Here's the drawing with two shaded views (mm, measured from the low corner). I have some questions. A direction names the side the tool comes from. Coordinates: 2 decimals unless noted, no trailing zeros. Write each loop counter-clockwise with the first axis right and the second up, starting at its lowest first coordinate (ties: lowest second). Pieces come first, ordered by that corner, then holes. Notation, with made-up numbers: (85, 27) -> (138, 27) arc R11 ccw to (138, 47) -> close; hole circle Ø1 at (43.5, 83.25). An arc over 180 degrees is marked (long way). Answer in a Markdown table with one row per item. Add a question column.
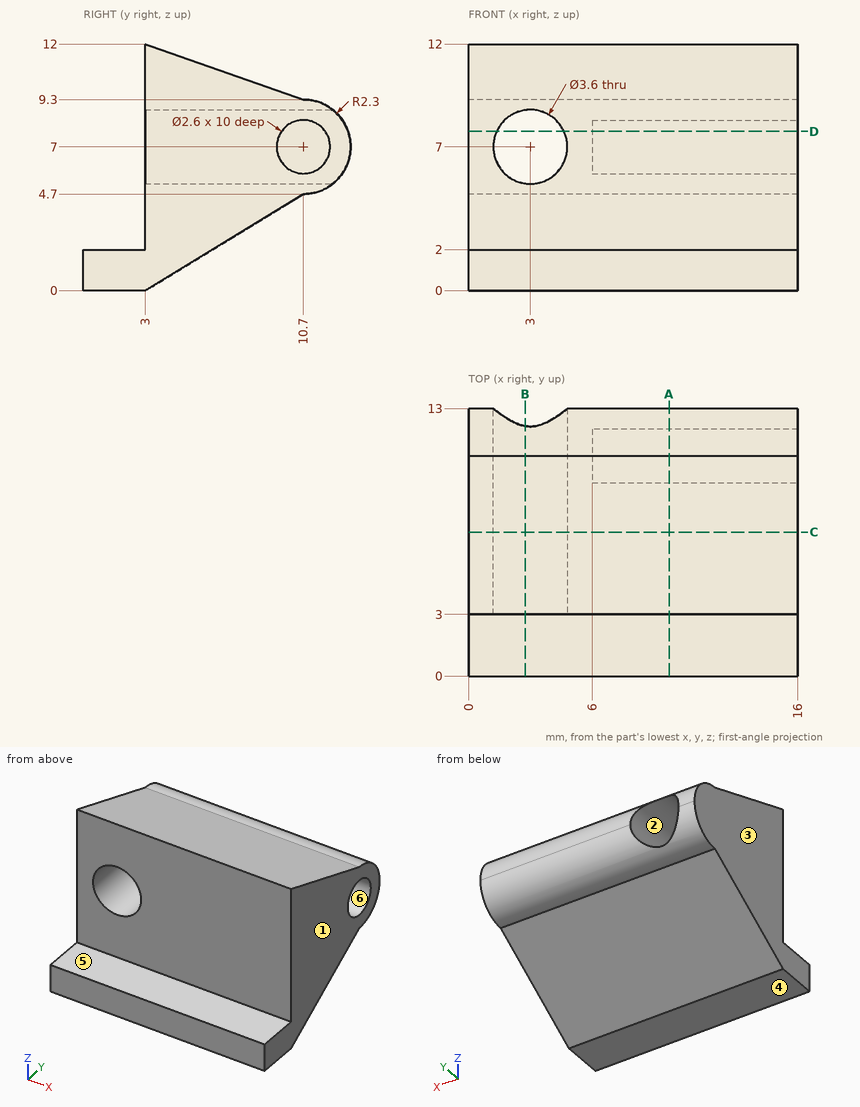
Q1. Imagine slicing it at C-C on y = 7. Please give me the cut outline in (x, z).
Q2. Imagine slicing it at B-B on x = 2.75. Please give me the cut outline in (y, z), plus the area to 3 significant figures.
Q3. I need wall thicknesses on line 1 (Z direction, x = 9.25, y = 10.7); line 2 (Z direction, x = 14.75, y = 1.25); line 3 (Y direction, x = 14.25, z = 6.25). Which ranges of each line are inside material? Lowest first, please. Write a range as [from, to].
Q4. I'm going to push flat-ended pins straight in: P1, Ø3, axis at x = 11.5, y = 2.5, coming from the +Z side; P2, Ø1.5, axis at y = 9, z = 1.5, coming from the -X side; P3, Ø2.5, axis at x = 9.5, y = 1.5, coming from the +Z side; P4, Ø3, axis at x = 8.5, z = 7.5, coming from the -Y side. Where does each tip first touch, or does it pass through?
Q5. If we mould it in two halves opening along X, with no side actions, what happens to the marked faces 1, 2 and 3? For each: pulls with the +X half, pulls with the -X half, needs draft (parallel to the pull), parting line crosses it, or undercut.
Q6. For the marked faces 4, 5 and 6, which set-ups out of +Z, -Z, +X, -X, +Y, -Y let a thin tool reach every point of the face, with its end or its side?
Q7. Imagine slicing it at A-A on x = 9.75. Please give me the cut outline in (y, z).
Q8. Imagine slicing it at D-D on z = 7.75. Please give me the cut outline in (x, y).
Result sheet:
| question | item | result |
|---|---|---|
| 1 | outline | (0, 2.44) -> (16, 2.44) -> (16, 10.6) -> (0, 10.6) -> close; hole circle Ø3.6 at (3, 7) |
| 2 | outline | (0, 0) -> (3, 0) -> (10.7, 4.7) arc R2.3 ccw to (12.15, 5.22) -> (3, 5.22) -> (3, 2) -> (0, 2) -> close; (3, 8.78) -> (12.15, 8.78) arc R2.3 ccw to (10.7, 9.3) -> (3, 12) -> close |
| 2 | area | 43.5 mm^2 |
| 3 | line 1 | z = [4.7, 5.7], [8.3, 9.3] |
| 3 | line 2 | z = [0, 2] |
| 3 | line 3 | y = [3, 9.64], [11.76, 12.87] |
| 4 | P1 | stops at z = 12 |
| 4 | P2 | passes through |
| 4 | P3 | stops at z = 2 |
| 4 | P4 | stops at y = 3 |
| 5 | face 1 | pulls with the +X half |
| 5 | face 2 | undercut |
| 5 | face 3 | pulls with the -X half |
| 6 | face 4 | -Z, +X, -X, +Y, -Y |
| 6 | face 5 | +Z, +X, -X, -Y |
| 6 | face 6 | +X |
| 7 | outline | (0, 0) -> (3, 0) -> (10.7, 4.7) arc R2.3 ccw to (10.7, 9.3) -> (3, 12) -> (3, 2) -> (0, 2) -> close; hole circle Ø2.6 at (10.7, 7) |
| 8 | outline | (0, 3) -> (1.36, 3) -> (1.36, 12.87) -> (0, 12.87) -> close; (4.64, 3) -> (16, 3) -> (16, 9.64) -> (6, 9.64) -> (6, 11.76) -> (16, 11.76) -> (16, 12.87) -> (4.64, 12.87) -> close |
